Part model, mm, in its own coordinate system. Face numbers are marked on the shaded views. Round coordinates to 2 decimals unless told otherwise and drop trailing zeros. Write each loop counter-clockwise with the first axis right and the second up, starting at its lowest first coordinate (ties: lowest second). Pieces come first, ordered by that corner, then holes. Notation, with made-up numbers: M -22.5,42 L 13.5,42 A18 cw 13.5,54 Z; hole C 16,69.5 d6. An arc over 180 degrees is marked long. Use one line per item in the form item = value. Start each with the question number.
Item 1: Cut at C-C, the plane z = 17.75. Give the cut face in (x, y), then the cut area to 3 significant figures.
Item 2: Probe L1, parallel to X at y = -2, z = 10; L2, parallel to Y at x = -61.5, z = 1.5; L3, parallel to X at y = 1.5, z = 6.25. List the from-to ranges inside material, lowest first.
Item 3: Cut at D-D, the plane x = -38. Give the cut face in (y, z), then the cut area to 3 significant figures.
Item 4: Mould opens along Y. For the marked faces 1, 2 and 3 say: +Y half, -Y half, draft (parallel to the pull), parting line (faces both ways), or undercut.
Item 5: Flat gauge pins, fed straight in: pin 1 Ø1.6 at (x, y) = (19.95, 0) entering from +Z; pin 2 Ø5 at (x, z) = (-35, 6) entering from +Y; pin 3 Ø5 at (x, z) = (-47, 21) entering from -Y; pin 4 Ø1 at (x, y) = (-42, 7.5) entering from -Z. Where does each tip first touch, or does it go through?
Item 6: Cut at B-B, the plane x = -61.5. Give the cut face in (y, z).
Item 7: Cut at A-A, the plane x = -97.5. Give the cut face in (y, z), then the cut area to 3 significant figures.
from build123d import *

# Parameters (mm, degrees)
REVOLVE1_ANGLE                  = 180
CUT_EXTRUDE3_START              = -2
SKETCH3_W                       = 60
SKETCH3_H                       = 25
CUT_EXTRUDE3_DEPTH              = 24
SKETCH7_R                       = 2
SKETCH7_W                       = 40
SKETCH7_H                       = 20
SKETCH7_R_2                     = 3
CUT_EXTRUDE8_DEPTH              = 10
CUT_EXTRUDE13_START             = 25
SKETCH16_R                      = 1
SKETCH16_W                      = 23.5
SKETCH16_H                      = 12.1
CUT_EXTRUDE13_DEPTH             = 23
CUT_EXTRUDE14_START             = -7
SKETCH18_W                      = 4.55
SKETCH18_H                      = 12.1
CUT_EXTRUDE14_DEPTH             = 19.0000001
SKETCH19_R                      = 2.5
CUT_EXTRUDE15_DEPTH             = 3
SKIZZE1_R                       = 4.489769008
SCHNITT_LINEAR_AUSTRAGEN1_DEPTH = 10
SKIZZE2_W                       = 23.5
SKIZZE2_H                       = 12.1
SCHNITT_LINEAR_AUSTRAGEN2_DEPTH = 10


with BuildPart() as part:
    # Sketch1 → Revolve1 (revolve)
    with BuildSketch(Plane.XY):
        with BuildLine():
            Line((-125, 0), (25, 0))
            ThreePointArc((25, 0), (17.67766953, 17.67766953), (0, 25))
            Line((0, 25), (-100, 25))
            ThreePointArc((-100, 25), (-117.67766953, 17.67766953), (-125, 0))
        make_face()
    revolve(axis=Axis((-125, 0, 0), (1, 0, 0)), revolution_arc=REVOLVE1_ANGLE)

    # Sketch3 → Cut-Extrude3 (cut, through all)
    with BuildSketch(Plane(origin=(0, 0, 0), x_dir=(-1, 0, 0), z_dir=(0, 0, -1)).offset(CUT_EXTRUDE3_START)):
        with Locations((85, 0)):
            Rectangle(SKETCH3_W, SKETCH3_H)
    extrude(amount=-CUT_EXTRUDE3_DEPTH, mode=Mode.SUBTRACT)

    # Sketch7 → Cut-Extrude8 (cut)
    with BuildSketch(Plane.XY.offset(2)):
        with Locations((-109.5, 5)):
            Circle(SKETCH7_R)
        with Locations((-61.5, 5)):
            Circle(SKETCH7_R)
        with Locations((-109.5, -5)):
            Circle(SKETCH7_R)
        with Locations((-61.5, -5)):
            Circle(SKETCH7_R)
        with Locations((-85.5, 0)):
            Rectangle(SKETCH7_W, SKETCH7_H)
        with Locations((-95.5, -0.25)):
            Circle(SKETCH7_R_2, mode=Mode.SUBTRACT)
    extrude(amount=-CUT_EXTRUDE8_DEPTH, mode=Mode.SUBTRACT)

    # Sketch16 → Cut-Extrude13 (cut)
    with BuildSketch(Plane.XY.offset(CUT_EXTRUDE13_START)):
        with Locations((-8.55, 0)):
            Circle(SKETCH16_R)
        with Locations((19.95, 0)):
            Circle(SKETCH16_R)
        with Locations((5.7, 0)):
            Rectangle(SKETCH16_W, SKETCH16_H)
    extrude(amount=-CUT_EXTRUDE13_DEPTH, mode=Mode.SUBTRACT)

    # Sketch18 → Cut-Extrude14 (cut, through all)
    with BuildSketch(Plane(origin=(0, 0, 0), x_dir=(-1, 0, 0), z_dir=(0, 0, -1)).offset(CUT_EXTRUDE14_START)):
        with Locations((-19.725, 0)):
            Rectangle(SKETCH18_W, SKETCH18_H)
        with Locations((8.325, 0)):
            Rectangle(SKETCH18_W, SKETCH18_H)
    extrude(amount=-CUT_EXTRUDE14_DEPTH, mode=Mode.SUBTRACT)

    # Sketch19 → Cut-Extrude15 (cut, through all)
    with BuildSketch(Plane.XY.offset(2)):
        with Locations((11, 0)):
            Circle(SKETCH19_R)
    extrude(amount=-CUT_EXTRUDE15_DEPTH, mode=Mode.SUBTRACT)

    # Skizze1 → Schnitt-Linear austragen1 (cut)
    with BuildSketch(Plane.XY.offset(2)):
        with Locations((-95.5, -0.25)):
            Circle(SKIZZE1_R)
    extrude(amount=-SCHNITT_LINEAR_AUSTRAGEN1_DEPTH, mode=Mode.SUBTRACT)

    # Skizze2 → Schnitt-Linear austragen2 (cut)
    with BuildSketch(Plane.XY.offset(2)):
        with Locations((5.7, 0)):
            Rectangle(SKIZZE2_W, SKIZZE2_H)
    extrude(amount=-SCHNITT_LINEAR_AUSTRAGEN2_DEPTH, mode=Mode.SUBTRACT)


solid = part.part
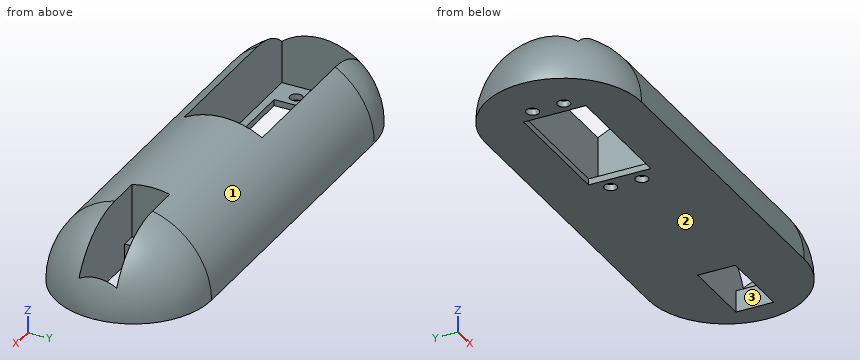
Model answer:
q1.outline = M -115,-9.22 L -115,9.22 A17.61 ccw Z; M -112.4,-12.5 A17.61 ccw -100,-17.61 L 0,-17.61 A17.61 ccw 16.53,-6.05 L -10.6,-6.05 L -10.6,6.05 L 16.53,6.05 A17.61 ccw 0,17.61 L -100,17.61 A17.61 ccw -112.4,12.5 L -55,12.5 L -55,-12.5 Z
q1.area = 2,670 mm²
q2.L1 = -122.83 to -115, -55 to -10.6, 22 to 22.83
q2.L2 = -24.95 to -7, -3 to 3, 7 to 24.95
q2.L3 = -124.16 to -115, -55 to -6.05, 17.45 to 24.16
q3.outline = M -25,0 L 25,0 A25 ccw Z
q3.area = 982 mm²
q4.face_1 = parting line
q4.face_2 = draft
q4.face_3 = undercut
q5.pin_1 = 2
q5.pin_2 = 24.75
q5.pin_3 = -16.82
q5.pin_4 = 0
q6.outline = M -25,0 L -7,0 L -7,2 L -12.5,2 L -12.5,21.65 A25 ccw Z; M -3,0 L 3,0 L 3,2 L -3,2 Z; M 7,0 L 25,0 A25 ccw 12.5,21.65 L 12.5,2 L 7,2 Z
q7.outline = M -25,0 L -10,0 L -10,2 L -12.5,2 L -12.5,21.65 A25 ccw Z; M 10,0 L 25,0 A25 ccw 12.5,21.65 L 12.5,2 L 10,2 Z
q7.area = 394 mm²
